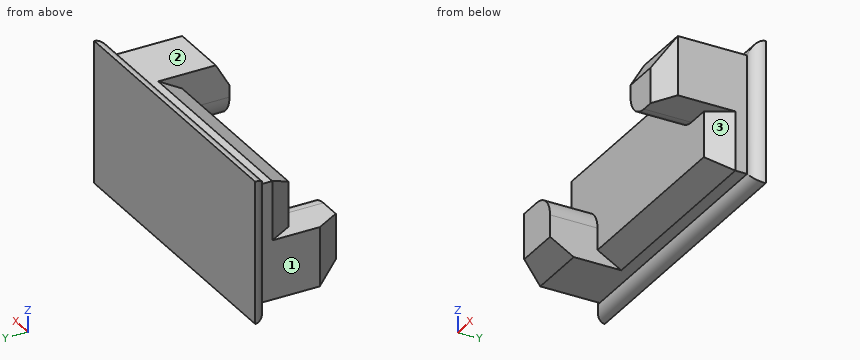
```python
from build123d import *

# Parameters (mm, degrees)
F1_DEPTH    = 25.4
F0_W        = 152.4
F0_H        = 76.2
F2_DEPTH    = 6.35
F3_DEPTH    = 50.8
F4_R        = 6.34999
F5_C1_SIZE2 = 7.3323484187
F5_C1_SIZE  = 12.7
F5_C2_SIZE2 = 7.3323484187
F5_C2_SIZE  = 12.7
F5_C3_SIZE2 = 12.7
F5_C3_SIZE  = 7.3323484187
F5_C4_SIZE2 = 7.3323484187
F5_C4_SIZE  = 12.7
F5_C5_SIZE2 = 7.3323484187
F5_C5_SIZE  = 12.7
F5_C6_SIZE2 = 12.7
F5_C6_SIZE  = 7.3323484187
F5_C7_SIZE2 = 7.3323484187
F5_C7_SIZE  = 12.7
F5_C8_SIZE2 = 7.3323484187
F5_C8_SIZE  = 12.7


# Not quite as in the source:
# - a fillet or chamfer is up to 0.001 mm smaller than in the source, because OpenCascade refuses the exact size


with BuildPart() as f1:
    # F0 (on Front) → F1 (new body)
    with BuildSketch(Plane.XZ):
        with BuildLine():
            Line((114.3, -6.35), (6.35, -6.35))
            Line((6.35, -6.35), (6.35, -38.1))
            Line((6.35, -38.1), (25.4, -38.1))
            ThreePointArc((25.4, -38.1), (34.3802561211, -41.8197438789), (38.1, -50.8))
            Line((38.1, -50.8), (38.1, -69.85))
            Line((38.1, -69.85), (146.05, -69.85))
            Line((146.05, -69.85), (146.05, -38.1))
            Line((146.05, -38.1), (127, -38.1))
            ThreePointArc((127, -38.1), (118.0197438789, -34.3802561211), (114.3, -25.4))
            Line((114.3, -25.4), (114.3, -6.35))
        make_face()
    extrude(amount=F1_DEPTH)

    # F0 (on Front) → F2 (join)
    with BuildSketch(Plane.XZ):
        with Locations((76.2, -38.1)):
            Rectangle(F0_W, F0_H)
        Polygon((6.35, -38.1), (6.35, -6.35), (114.3, -6.35), (146.05, -6.35), (146.05, -38.1), (146.05, -69.85), (38.1, -69.85), (6.35, -69.85), align=None, mode=Mode.SUBTRACT)
    extrude(amount=F2_DEPTH)

    # F0 (on Front) → F3 (join)
    with BuildSketch(Plane.XZ):
        with BuildLine():
            Line((25.4, -38.1), (6.35, -38.1))
            Line((6.35, -38.1), (6.35, -69.85))
            Line((6.35, -69.85), (38.1, -69.85))
            Line((38.1, -69.85), (38.1, -50.8))
            ThreePointArc((38.1, -50.8), (34.3802561211, -41.8197438789), (25.4, -38.1))
        make_face()
        with BuildLine():
            Line((146.05, -6.35), (114.3, -6.35))
            Line((114.3, -6.35), (114.3, -25.4))
            ThreePointArc((114.3, -25.4), (118.0197438789, -34.3802561211), (127, -38.1))
            Line((127, -38.1), (146.05, -38.1))
            Line((146.05, -38.1), (146.05, -6.35))
        make_face()
    extrude(amount=F3_DEPTH)

    # F4 (radius 6.35 in the source; OpenCascade refuses exactly that, so slightly less here)
    f4_edges = [f1.edges().sort_by_distance(p)[0] for p in [
        (76.2, -6.35, -76.2),
        (0, -6.35, -38.1),
        (152.4, -6.35, -38.1),
        (76.2, -6.35, 0),
    ]]
    fillet(f4_edges, radius=F4_R)

    # F5: chamfer of 12.7 x 7.3323484187 on 8 edges, made by hand

    # F5_c1
    f5_c1_edges = [f1.edges().sort_by_distance(p)[0] for p in [
        (6.35, -25.4, -22.225),
    ]]
    f5_c1_side = f1.faces().sort_by_distance((6.35, -25.2533530316, -22.225))[0]
    chamfer(f5_c1_edges, length=F5_C1_SIZE, length2=F5_C1_SIZE2, reference=f5_c1_side)

    # F5_c2
    f5_c2_edges = [f1.edges().sort_by_distance(p)[0] for p in [
        (6.35, -50.8, -53.975),
    ]]
    f5_c2_side = f1.faces().sort_by_distance((6.35, -50.6533530316, -53.975))[0]
    chamfer(f5_c2_edges, length=F5_C2_SIZE, length2=F5_C2_SIZE2, reference=f5_c2_side)

    # F5_c3
    f5_c3_edges = [f1.edges().sort_by_distance(p)[0] for p in [
        (130.175, -50.8, -6.35),
    ]]
    f5_c3_side = f1.faces().sort_by_distance((130.175, -50.6533530316, -6.35))[0]
    chamfer(f5_c3_edges, length=F5_C3_SIZE, length2=F5_C3_SIZE2, reference=f5_c3_side)

    # F5_c4
    f5_c4_edges = [f1.edges().sort_by_distance(p)[0] for p in [
        (63.9911742094, -25.4, -6.35),
    ]]
    f5_c4_side = f1.faces().sort_by_distance((63.9911742094, -25.2533530316, -6.35))[0]
    chamfer(f5_c4_edges, length=F5_C4_SIZE, length2=F5_C4_SIZE2, reference=f5_c4_side)

    # F5_c5
    f5_c5_edges = [f1.edges().sort_by_distance(p)[0] for p in [
        (146.05, -25.4, -53.975),
    ]]
    f5_c5_side = f1.faces().sort_by_distance((146.05, -25.2533530316, -53.975))[0]
    chamfer(f5_c5_edges, length=F5_C5_SIZE, length2=F5_C5_SIZE2, reference=f5_c5_side)

    # F5_c6
    f5_c6_edges = [f1.edges().sort_by_distance(p)[0] for p in [
        (146.05, -50.8, -28.575),
    ]]
    f5_c6_side = f1.faces().sort_by_distance((146.05, -50.6533530316, -28.575))[0]
    chamfer(f5_c6_edges, length=F5_C6_SIZE, length2=F5_C6_SIZE2, reference=f5_c6_side)

    # F5_c7
    f5_c7_edges = [f1.edges().sort_by_distance(p)[0] for p in [
        (25.8911742094, -50.8, -69.85),
    ]]
    f5_c7_side = f1.faces().sort_by_distance((25.8911742094, -50.6533530316, -69.85))[0]
    chamfer(f5_c7_edges, length=F5_C7_SIZE, length2=F5_C7_SIZE2, reference=f5_c7_side)

    # F5_c8
    f5_c8_edges = [f1.edges().sort_by_distance(p)[0] for p in [
        (88.4088257906, -25.4, -69.85),
    ]]
    f5_c8_side = f1.faces().sort_by_distance((88.4088257906, -25.2533530316, -69.85))[0]
    chamfer(f5_c8_edges, length=F5_C8_SIZE, length2=F5_C8_SIZE2, reference=f5_c8_side)


solid = f1.part
```
Build history of the part. All positions in model axes, mm. Face numbers are marked on the shaded views. A direction names the side the tool comes from. Round coordinates to 2 decimals unless told otherwise and drop trailing zeros. Write each loop counter-clockwise with the first axis right and the second up, starting at its lowest first coordinate (ties: lowest second). Pieces come first, ordered by that corner, then holes.
1) Band-saw the part on A-A, the plane y = -29. List the corners of the cut face in (x, z), and give its area (3 significant figures).
2) Drill centre lines: probe 1 along Y at (x, z) = (66, -46.5); probe 2 along X at (y, z) = (-9.5, -15); probe 3 along X at (y, z) = (-34, -25). Where is each one in solid material? Low to high.
3) Pin check, flat tips, straight feed: pin 1 (19 mm diameter, centred on x = 64, z = -51, fed in from -Y); pin 2 (18.5 mm diameter, centred on x = 110.5, y = -32, fed in from +Z); pin 3 (15 mm diameter, centred on y = -39, z = -64.5, fed in from +X); pin 4 (12 mm diameter, centred on y = -5.5, z = -54.5, fed in from -X). Stop position of each tip, or through.
4) 3-axis set-ups, long thin cutter, end or side, ignore diameter. For the marked faces 1, 2 and 3: which of +Z, -Z, +X, -X, +Y, -Y reach the whole face in a straight line?
Ans:
1. outline: (6.35, -69.85) - (38.1, -69.85) - (38.1, -50.8) arc R12.7 ccw to (25.4, -38.1) - (6.35, -38.1) - close; (114.3, -25.4) arc R12.7 ccw to (127, -38.1) - (146.05, -38.1) - (146.05, -6.35) - (114.3, -6.35) - close
1. area: 1,950 mm2
2. probe 1: y = -25.4 to 0
2. probe 2: x = 6.35 to 146.05
2. probe 3: x = 114.3 to 146.05
3. pin 1: stops at y = -25.4
3. pin 2: stops at z = -6.35
3. pin 3: stops at x = 38.1
3. pin 4: stops at x = 0
4. face 1: +Z, -Z, -X, -Y
4. face 2: +Z, +X, -X, -Y
4. face 3: -Z, +X, -Y
